Source: CAD feature listing. Evaluate the final solid. Frame: model axes, mm. A direction names the side the tool comes from. Give positions to 0.01 mm unless a question says otherwise; leave off trailing zeros. Write each loop counter-clockwise with the first axis right and the second up, starting at its lowest first coordinate (ties: lowest second). Pieces come first, ordered by that corner, then holes. Notation, with made-up numbers: (-3.5, -40) -> (51.5, -40) arc R31 cw to (51.5, -14) -> close; hole circle Ø7 at (45, 22.25). An arc over 180 degrees is marked (long way). Write item = value, one per line.
from build123d import *

# Parameters (mm, degrees)
SKETCH1_W           = 50
SKETCH1_H           = 50
SKETCH1_R           = 5
BOSS_EXTRUDE1_DEPTH = 2.5
SKETCH2_W           = 5
SKETCH2_H           = 15
BOSS_EXTRUDE2_DEPTH = 15
SKETCH3_R           = 2.5
CUT_EXTRUDE1_DEPTH  = 47.435439053
FILLET1_R           = 7.5


with BuildPart() as part:
    # Sketch1 → Boss-Extrude1 (new body)
    with BuildSketch(Plane.XY):
        Rectangle(SKETCH1_W, SKETCH1_H)
        with Locations((17.67766953, 17.67766953)):
            Circle(SKETCH1_R, mode=Mode.SUBTRACT)
        with Locations(Location((-17.67766953, 17.67766953, 0), (0, 0, 180))):
            Circle(SKETCH1_R, mode=Mode.SUBTRACT)
        with Locations(Location((17.67766953, -17.67766953, 0), (0, 0, 180))):
            Circle(SKETCH1_R, mode=Mode.SUBTRACT)
        with Locations((-17.67766953, -17.67766953)):
            Circle(SKETCH1_R, mode=Mode.SUBTRACT)
    extrude(amount=BOSS_EXTRUDE1_DEPTH)

    # Sketch2 → Boss-Extrude2 (add)
    with BuildSketch(Plane.XY.offset(2.5)):
        with Locations((-7.5, 0)):
            Rectangle(SKETCH2_W, SKETCH2_H)
        with Locations((7.5, 0)):
            Rectangle(SKETCH2_W, SKETCH2_H)
    extrude(amount=BOSS_EXTRUDE2_DEPTH)

    # Sketch3 → Cut-Extrude1 (cut, through all)
    with BuildSketch(Plane(origin=(10, 0, 0), x_dir=(0, 0, -1), z_dir=(1, 0, 0))):
        with Locations((-10, 0)):
            Circle(SKETCH3_R)
    extrude(amount=-CUT_EXTRUDE1_DEPTH, mode=Mode.SUBTRACT)

    # Fillet1
    fillet1_edges = [part.edges().sort_by_distance(p)[0] for p in [
        (-7.5, 7.5, 17.5),
        (-7.5, -7.5, 17.5),
        (7.5, -7.5, 17.5),
        (7.5, 7.5, 17.5),
    ]]
    fillet(fillet1_edges, radius=FILLET1_R - 0.0001)  # a hair under: the kernel refuses the full size


solid = part.part
1) Draft query along X for faces 1 (the flat face through (25, 0, 1)), 2 (the flat face through (-10, -2, 8)), 3 (the flat face through (5, -2, 8)). Return one class per face: pulls with the +X half, pulls with the -X half, needs draft (parallel to the pull), parting line crosses it, or undercut.
Computed:
face_1 = pulls with the +X half
face_2 = pulls with the -X half
face_3 = undercut
2) Contact query for flat-ended pins moving along their axis: pin 1 (7.5 mm diameter, centred on y = -3.5, z = 7, fed in from -X); pin 2 (2.5 mm diameter, centred on x = 6.5, z = 7.5, fed in from -Y); pin 3 (13 mm diameter, centred on x = -17.68, y = -17.68, fed in from +Z). Output: stop coordinate, or through.
Computed:
pin_1 = -10
pin_2 = -7.5
pin_3 = 2.5
3) Access query for faces 4 (the flat face through (-5, -2, 8)), 5 (the flat face through (7, -7.5, 6)), 6 (the flat face through (10, -2, 8)). Directions: +Z, -Z, +X, -X, +Y, -Y. A direction counts if a zero-diameter tool reaches every point of the face in a straight line with its end or side. Return the directions, or none.
Computed:
face_4 = +Z, +Y, -Y
face_5 = +Z, +X, -X, -Y
face_6 = +Z, +X, +Y, -Y
4) Cut plane C-C (z = 3.75). Return the cut outline in (x, y).
Computed:
outline = (-10, -7.5) -> (-5, -7.5) -> (-5, 7.5) -> (-10, 7.5) -> close; (5, -7.5) -> (10, -7.5) -> (10, 7.5) -> (5, 7.5) -> close
5) Cut plane D-D (z = 9.25). Return the cut outline in (x, y).
Computed:
outline = (-10, -7.5) -> (-5, -7.5) -> (-5, -2.38) -> (-10, -2.38) -> close; (-10, 2.38) -> (-5, 2.38) -> (-5, 7.5) -> (-10, 7.5) -> close; (5, -7.5) -> (10, -7.5) -> (10, -2.38) -> (5, -2.38) -> close; (5, 2.38) -> (10, 2.38) -> (10, 7.5) -> (5, 7.5) -> close
6) Cut plane B-B (y = 20). Return the cut outline in (x, z).
Computed:
outline = (-25, 0) -> (-22.11, 0) -> (-22.11, 2.5) -> (-25, 2.5) -> close; (-13.25, 0) -> (13.25, 0) -> (13.25, 2.5) -> (-13.25, 2.5) -> close; (22.11, 0) -> (25, 0) -> (25, 2.5) -> (22.11, 2.5) -> close
7) Material intervals for L1, parallel to X at y = -3, z = 6.75; L2, parallel to Y at x = -7.75, z = 10; L3, parallel to Z at x = 8, y = -17, sorted ascending.
Computed:
L1 = -10 to -5, 5 to 10
L2 = -7.5 to -2.5, 2.5 to 7.5
L3 = 0 to 2.5
